Autodesk Inventor part; units mm, degrees
ref_plane "YZ Plane" through (0, 0, 0) normal (1, 0, 0) x (0, 1, 0)
ref_plane "XZ Plane" through (0, 0, 0) normal (0, 1, 0) x (-1, 0, 0)
ref_plane "XY Plane" through (0, 0, 0) normal (0, 0, 1) x (1, 0, 0)
sketch "Sketch1" plane through (0, 0, 0) normal (0, 0, 1) x (1, 0, 0)
  circle A0 centre (0, 0) radius 1
  dimension "d0" = 2
extrude "Extrusion1" add sketch "Sketch1" along normal blind 12
thread "Thread1"
sketch "Sketch2" plane through (0, 0, 12) normal (0, 0, 1) x (1, 0, 0)
  circle A0 centre (0, 0) radius 1
  circle A1 centre (0, 0) radius 1.85
  dimension "d6" = 3.7
extrude "Extrusion2" add sketch "Sketch2" along normal blind 1.7 contours A0 | A1
fillet "Fillet1" radius 0.8 1 edges at (-1.85, 0, 13.7)
sketch "Sketch3" plane through (0, 0, 13.7) normal (0, 0, 1) x (1, 0, 0)
  circle A0 centre (0, 0) radius 1.05
  line L0 (-0.35, 1.25) -> (0.35, 1.25)
  line L1 (0.35, 1.25) -> (0.35, -1.25)
  line L2 (0.35, -1.25) -> (-0.35, -1.25)
  line L3 (-0.35, -1.25) -> (-0.35, 1.25)
  line L4 (-1.25, 0.35) -> (1.25, 0.35)
  line L5 (1.25, 0.35) -> (1.25, -0.35)
  line L6 (1.25, -0.35) -> (-1.25, -0.35)
  line L7 (-1.25, -0.35) -> (-1.25, 0.35)
  point P0 (0, 1.25)
  point P1 (0.35, 0)
  point P2 (-1.25, 0)
  point P3 (0, 0.35)
  dimension "d11" = 0.7
  dimension "d15" = 2.5
  dimension "d16" = 0.7
  dimension "d17" = 2.5
extrude "Extrusion3" cut sketch "Sketch3" against normal blind 1 contours A0 L6 L1 L4 | A0 L4 L5 L6 | L1 L4 L3 A0 | A0 L3 L0 L1 | L1 L6 L3 L4 | L1 L2 L3 A0 | A0 L3 L6 L1 | L3 L6 A0 L4 | A0 L6 L7 L4
equation "\"d16\" = d11"
equation "\"d17\" = d15"
properties part number "M2 Screw"
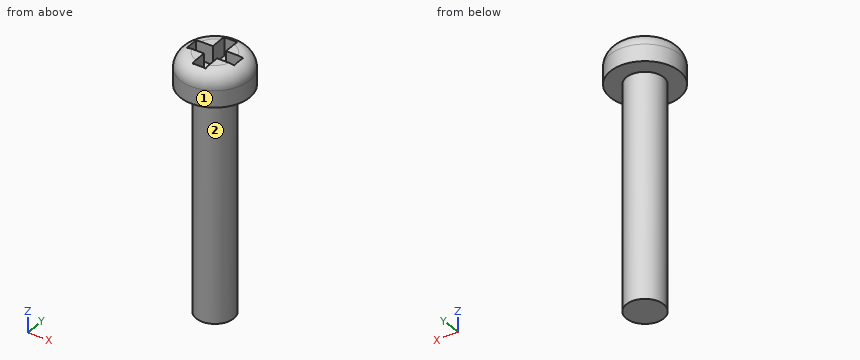
Geometry: final body of the model. Coordinates: model frame, mm. Face numbers are marked on the shaded views. A direction names the side the tool comes from. Coordinates: 2 decimals unless noted, no trailing zeros. Order: outer loops, then holes, each group sorted by start corner. A loop starts at its lowest first (then second) coordinate and runs counter-clockwise, first axis right, second up. Notation, with made-up numbers: (74.5, 36) - (84.5, 36) arc R11 cw to (84.5, 41) - close; hole circle Ø1 at (23.5, 68.25). An arc over 180 degrees is marked (long way). Return JSON: item names as keys, results as strings. Group by question number.
1. Pin query (flat end, axial travel): pin 1 (0.8 mm diameter, centred on x = 0, z = 13.5, fed in from +Y); pin 2 (0.5 mm diameter, centred on x = 1, z = 13.5, fed in from +Y); pin 3 (1 mm diameter, centred on x = 1, z = 13.5, fed in from -Y). Return the tip coordinate at first contact, or that it passes through.
2. Cut plane C-C (z = 6.5). Output: boundary loops of the cut face in (x, y), plus the area to 3 significant figures.
3. Set-up query: the marked faces 1 and 2. Return all of +Z, -Z, +X, -X, +Y, -Y with unobstructed straight access to the full face (end or side cutting, diameter ignored); none if empty.
4. Material intervals for line 1 along Z through (x, y) = (1.1, 0.6); line 2 along Z through (x, y) = (1.1, -0.25); line 3 along X through (y, z) = (-0.1, 5.75), sorted ascending. Write a range as [from, to].
5. Cut plane A-A (y = 0). Output: boundary loops of the cut face in (x, z).
Resolved:
{
 "1": {"pin 1": "stops at y = 1.82", "pin 2": "stops at y = 1.52", "pin 3": "stops at y = -1.69"},
 "2": {"outline": "circle Ø2 at (0, 0)", "area": "3.14 mm²"},
 "3": {"face 1": "+Z, -Z", "face 2": "-Z"},
 "4": {"line 1": "z = [12, 13.67]", "line 2": "z = [12, 12.7]", "line 3": "x = [-0.99, 0.99]"},
 "5": {"outline": "(-1.85, 12) - (-1, 12) - (-1, 0) - (1, 0) - (1, 12) - (1.85, 12) - (1.85, 12.9) arc R0.8 ccw to (1.25, 13.67) - (1.25, 12.7) - (-1.25, 12.7) - (-1.25, 13.67) arc R0.8 ccw to (-1.85, 12.9) - close"}
}
